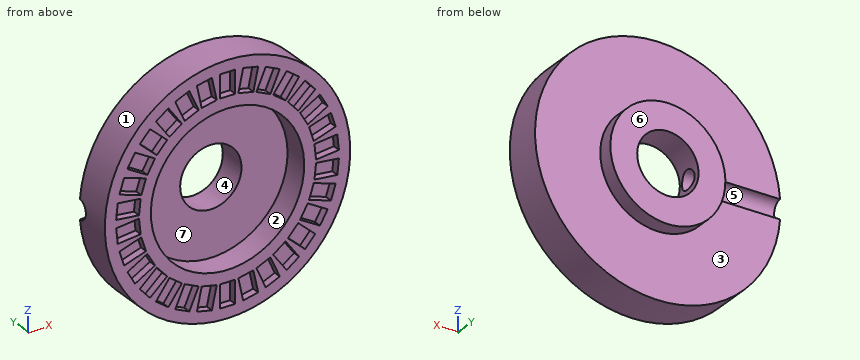
from build123d import *

# Parameters (mm, degrees)
SKETCH1_R           = 16
SKETCH1_W           = 2
SKETCH1_H           = 3
SKETCH1_R_2         = 10
BOSS_EXTRUDE3_DEPTH = 1
SKETCH2_R           = 16
SKETCH2_R_2         = 10
BOSS_EXTRUDE4_DEPTH = 1.5
SKETCH3_R           = 16
SKETCH3_R_2         = 10
BOSS_EXTRUDE5_DEPTH = 0.8
SKETCH4_R           = 16
BOSS_EXTRUDE6_DEPTH = 1.7
SKETCH5_R           = 4
CUT_EXTRUDE3_DEPTH  = 1.7
BOSS_EXTRUDE8_START = 2
SKETCH6_R           = 7.5
SKETCH6_R_2         = 4
BOSS_EXTRUDE8_DEPTH = 2
SKETCH8_R           = 1.25
CUT_EXTRUDE5_DEPTH  = 29


with BuildPart() as part:
    # Sketch1 → Boss-Extrude3 (new body)
    with BuildSketch(Plane(origin=(0, 0, 0), x_dir=(1, 0, 0), z_dir=(0, 1, 0))):
        with Locations(Location((0, 0, 0), (0, 0, 270))):
            Circle(SKETCH1_R)
        Polygon((3.992867118, 13.97522852), (3.369132045, 11.040785718), (1.412836844, 11.456609099), (2.036571916, 14.391051901), align=None, mode=Mode.SUBTRACT)
        with Locations((0, 13)):
            Rectangle(SKETCH1_W, SKETCH1_H, mode=Mode.SUBTRACT)
        Polygon((6.811226782, 12.839672493), (5.591016853, 10.09903612), (3.763925938, 10.912509406), (4.984135867, 13.653145779), align=None, mode=Mode.SUBTRACT)
        Polygon((-2.036571916, 14.391051901), (-1.412836844, 11.456609099), (-3.369132045, 11.040785718), (-3.992867118, 13.97522852), align=None, mode=Mode.SUBTRACT)
        Polygon((9.331903153, 11.142961166), (7.568547396, 8.715910183), (5.950513407, 9.891480688), (7.713869164, 12.318531671), align=None, mode=Mode.SUBTRACT)
        Polygon((-4.984135867, 13.653145779), (-3.763925938, 10.912509406), (-5.591016853, 10.09903612), (-6.811226782, 12.839672493), align=None, mode=Mode.SUBTRACT)
        Polygon((-9.331903153, -11.142961166), (-7.568547396, -8.715910183), (-5.950513407, -9.891480688), (-7.713869164, -12.318531671), align=None, mode=Mode.SUBTRACT)
        Polygon((-11.444730576, -8.959248967), (-9.215296099, -6.951857148), (-7.877034887, -8.438146799), (-10.106469363, -10.445538618), align=None, mode=Mode.SUBTRACT)
        Polygon((-6.811226782, -12.839672493), (-5.591016853, -10.09903612), (-3.763925938, -10.912509406), (-4.984135867, -13.653145779), align=None, mode=Mode.SUBTRACT)
        with Locations((0, -13)):
            Rectangle(SKETCH1_W, SKETCH1_H, mode=Mode.SUBTRACT)
        Polygon((-1.412836844, -11.456609099), (-2.036571916, -14.391051901), (-3.992867118, -13.97522852), (-3.369132045, -11.040785718), align=None, mode=Mode.SUBTRACT)
        Polygon((-13.057368355, -6.383974596), (-10.459292144, -4.883974596), (-9.459292144, -6.616025404), (-12.057368355, -8.116025404), align=None, mode=Mode.SUBTRACT)
        Polygon((-14.099336481, -3.529689902), (-11.246166932, -2.602638919), (-10.628132943, -4.504751952), (-13.481302492, -5.431802935), align=None, mode=Mode.SUBTRACT)
        Polygon((-14.525095946, -0.521140822), (-11.54153026, -0.207555432), (-11.332473333, -2.196599223), (-14.31603902, -2.510184613), align=None, mode=Mode.SUBTRACT)
        Polygon((2.036571916, -14.391051901), (1.412836844, -11.456609099), (3.369132045, -11.040785718), (3.992867118, -13.97522852), align=None, mode=Mode.SUBTRACT)
        Polygon((4.984135867, -13.653145779), (3.763925938, -10.912509406), (5.591016853, -10.09903612), (6.811226782, -12.839672493), align=None, mode=Mode.SUBTRACT)
        Polygon((7.713869164, -12.318531671), (5.950513407, -9.891480688), (7.568547396, -8.715910183), (9.331903153, -11.142961166), align=None, mode=Mode.SUBTRACT)
        Polygon((10.106469363, -10.445538618), (7.877034887, -8.438146799), (9.215296099, -6.951857148), (11.444730576, -8.959248967), align=None, mode=Mode.SUBTRACT)
        Polygon((12.057368355, -8.116025404), (9.459292144, -6.616025404), (10.459292144, -4.883974596), (13.057368355, -6.383974596), align=None, mode=Mode.SUBTRACT)
        Polygon((13.481302492, -5.431802935), (10.628132943, -4.504751952), (11.246166932, -2.602638919), (14.099336481, -3.529689902), align=None, mode=Mode.SUBTRACT)
        Polygon((14.31603902, -2.510184613), (11.332473333, -2.196599223), (11.54153026, -0.207555432), (14.525095946, -0.521140822), align=None, mode=Mode.SUBTRACT)
        Polygon((-14.31603902, 2.510184613), (-11.332473333, 2.196599223), (-11.54153026, 0.207555432), (-14.525095946, 0.521140822), align=None, mode=Mode.SUBTRACT)
        Polygon((-13.481302492, 5.431802935), (-10.628132943, 4.504751952), (-11.246166932, 2.602638919), (-14.099336481, 3.529689902), align=None, mode=Mode.SUBTRACT)
        with Locations(Location((0, 0, 0), (0, 0, 270))):
            Circle(SKETCH1_R_2, mode=Mode.SUBTRACT)
        Polygon((-12.057368355, 8.116025404), (-9.459292144, 6.616025404), (-10.459292144, 4.883974596), (-13.057368355, 6.383974596), align=None, mode=Mode.SUBTRACT)
        Polygon((-10.106469363, 10.445538618), (-7.877034887, 8.438146799), (-9.215296099, 6.951857148), (-11.444730576, 8.959248967), align=None, mode=Mode.SUBTRACT)
        Polygon((-7.713869164, 12.318531671), (-5.950513407, 9.891480688), (-7.568547396, 8.715910183), (-9.331903153, 11.142961166), align=None, mode=Mode.SUBTRACT)
        Polygon((14.525095946, 0.521140822), (11.54153026, 0.207555432), (11.332473333, 2.196599223), (14.31603902, 2.510184613), align=None, mode=Mode.SUBTRACT)
        Polygon((14.099336481, 3.529689902), (11.246166932, 2.602638919), (10.628132943, 4.504751952), (13.481302492, 5.431802935), align=None, mode=Mode.SUBTRACT)
        Polygon((7.877034887, 8.438146799), (10.106469363, 10.445538618), (11.444730576, 8.959248967), (9.215296099, 6.951857148), align=None, mode=Mode.SUBTRACT)
        Polygon((13.057368355, 6.383974596), (10.459292144, 4.883974596), (9.459292144, 6.616025404), (12.057368355, 8.116025404), align=None, mode=Mode.SUBTRACT)
    extrude(amount=BOSS_EXTRUDE3_DEPTH)

    # Sketch2 → Boss-Extrude4 (add)
    with BuildSketch(Plane(origin=(0, 1, 0), x_dir=(1, 0, 0), z_dir=(0, 1, 0))):
        with Locations(Location((0, 0, 0), (0, 0, 270))):
            Circle(SKETCH2_R)
        with Locations(Location((0, 0, 0), (0, 0, 270))):
            Circle(SKETCH2_R_2, mode=Mode.SUBTRACT)
    extrude(amount=BOSS_EXTRUDE4_DEPTH)

    # Sketch3 → Boss-Extrude5 (add)
    with BuildSketch(Plane(origin=(0, 2.5, 0), x_dir=(1, 0, 0), z_dir=(0, 1, 0))):
        with Locations(Location((0, 0, 0), (0, 0, 270))):
            Circle(SKETCH3_R)
        with Locations(Location((0, 0, 0), (0, 0, 270))):
            Circle(SKETCH3_R_2, mode=Mode.SUBTRACT)
    extrude(amount=BOSS_EXTRUDE5_DEPTH)

    # Sketch4 → Boss-Extrude6 (add)
    with BuildSketch(Plane(origin=(0, 3.3, 0), x_dir=(1, 0, 0), z_dir=(0, 1, 0))):
        with Locations(Location((0, 0, 0), (0, 0, 270))):
            Circle(SKETCH4_R)
    extrude(amount=BOSS_EXTRUDE6_DEPTH)

    # Sketch5 → Cut-Extrude3 (cut)
    with BuildSketch(Plane(origin=(0, 5, 0), x_dir=(1, 0, 0), z_dir=(0, 1, 0))):
        with Locations(Location((0, 0, 0), (0, 0, 270))):
            Circle(SKETCH5_R)
    extrude(amount=-CUT_EXTRUDE3_DEPTH, mode=Mode.SUBTRACT)

    # Sketch6 → Boss-Extrude8 (add)
    with BuildSketch(Plane(origin=(0, 5, 0), x_dir=(1, 0, 0), z_dir=(0, 1, 0)).offset(BOSS_EXTRUDE8_START)):
        with Locations(Location((0, 0, 0), (0, 0, 270))):
            Circle(SKETCH6_R)
        with Locations(Location((0, 0, 0), (0, 0, 270))):
            Circle(SKETCH6_R_2, mode=Mode.SUBTRACT)
    extrude(amount=-BOSS_EXTRUDE8_DEPTH)

    # Sketch8 → Cut-Extrude5 (cut)
    with BuildSketch(Plane(origin=(0, 0, 0), x_dir=(0, 0, -1), z_dir=(1, 0, 0))):
        with Locations((0, 5)):
            Circle(SKETCH8_R)
    extrude(amount=-CUT_EXTRUDE5_DEPTH, mode=Mode.SUBTRACT)


solid = part.part
Build history of the part. All positions in model axes, mm. Face numbers are marked on the shaded views. A direction names the side the tool comes from. Give positions to 0.01 mm unless a question says otherwise; leave off trailing zeros. Order: outer loops, then holes, each group sorted by start corner. A loop starts at its lowest first (then second) coordinate and runs counter-clockwise, first axis right, second up. Notation, with made-up numbers: M 82,-25 L 111,-25 A20 cw 111,3 Z; hole C 49.25,-40 d4. An arc over 180 degrees is marked long. Put each result on its own line as item: value.
Item 1: Slice it at A-A, the plane x = 0. Write the cut outline in (y, z).
From the geometry:
outline: M 0,-16 L 5,-16 L 5,-7.5 L 7,-7.5 L 7,-4 L 3.3,-4 L 3.3,-10 L 0,-10 L 0,-11.5 L 1,-11.5 L 1,-14.5 L 0,-14.5 Z; M 0,10 L 3.3,10 L 3.3,4 L 7,4 L 7,7.5 L 5,7.5 L 5,16 L 0,16 L 0,14.5 L 1,14.5 L 1,11.5 L 0,11.5 Z
Item 2: 3-axis set-ups, long thin cutter, end or side, ignore diameter. For the marked faces 5, 6 and 7: which of +Z, -Z, +X, -X, +Y, -Y reach the whole face in a straight line?
From the geometry:
face 5: -X
face 6: +Z, -Z, +X, -X, +Y
face 7: -Y
Item 3: Slice it at B-B, the plane y = 2. Write the cut outline in (x, z).
From the geometry:
outline: C 0,0 d32; hole C 0,0 d20
Item 4: Flat gauge pins, fed straight in: pin 1 Ø2.5 at (x, z) = (8, -11) entering from -Y; pin 2 Ø2 at (x, y) = (-10, 1.5) entering from -Z; pin 3 Ø1.5 at (y, z) = (3, -11.5) entering from -X; pin 4 Ø1.1 at (y, z) = (0.5, 12.5) entering from +X. Where does each tip first touch, or does it go through?
From the geometry:
pin 1: stops at y = 0
pin 2: stops at z = -13.23
pin 3: stops at x = -11.85
pin 4: stops at x = 10.64
Item 5: Slice it at C-C, the plane y = 4.5. Write the cut outline in (x, z), plus the area to 3 significant figures.
From the geometry:
outline: M -15.96,-1.15 A16 ccw long -15.96,1.15 L -3.83,1.15 A4 cw long -3.83,-1.15 Z
area: 726 mm2
Item 6: Probe line 1 (X direction, y = 1.7, z = 0); line 2 (Y direction, x = -6.25, z = 0); line 3 (Z direction, x = -6, y = 4.5). List the from-to ranges inside material, lowest first. Write a range as [from, to].
From the geometry:
line 1: x = [-16, -10], [10, 16]
line 2: y = [3.3, 3.75], [6.25, 7]
line 3: z = [-14.83, -1.15], [1.15, 14.83]
Item 7: Two-plate mould, pull along X, no slides. Class the marked faces 1, 2, 3 and 4: +X half, -X half, draft (parallel to the pull), parting line (faces both ways), or undercut.
From the geometry:
face 1: parting line
face 2: undercut
face 3: draft
face 4: undercut
